from build123d import *

# Parameters (mm, degrees)
SKETCH1_W           = 292.1
SKETCH1_H           = 101.0158
SKETCH1_W_2         = 6.35
SKETCH1_H_2         = 7.62
BOSS_EXTRUDE1_DEPTH = 6
SKETCH2_R           = 11.125
SKETCH2_R_2         = 1.5875
SKETCH2_R_3         = 1.4605
CUT_EXTRUDE1_DEPTH  = 310.132013628
SKETCH3_W           = 7.62
SKETCH3_H           = 6
CUT_EXTRUDE2_DEPTH  = 310.132013628
SKETCH4_W           = 7.62
SKETCH4_H           = 0.35
CUT_EXTRUDE3_DEPTH  = 6
FILLET1_R           = 2.54
SKETCH5_R           = 1.143
CUT_EXTRUDE4_DEPTH  = 310.132013628
SKETCH6_R           = 1.905
SKETCH6_W           = 6.35
SKETCH6_H           = 7.62
CUT_EXTRUDE5_DEPTH  = 310.132013628
SKETCH7_R           = 1.8034
CUT_EXTRUDE6_DEPTH  = 310.132013628
SKETCH8_R           = 1.5875
CUT_EXTRUDE7_DEPTH  = 310.132013628


with BuildPart() as part:
    # Sketch1 → Boss-Extrude1 (new body)
    with BuildSketch(Plane.XY):
        with Locations((146.05, 50.5079)):
            Rectangle(SKETCH1_W, SKETCH1_H)
        with Locations((231.775, 93.7514)):
            Rectangle(SKETCH1_W_2, SKETCH1_H_2, mode=Mode.SUBTRACT)
        with Locations((73.025, 93.7514)):
            Rectangle(SKETCH1_W_2, SKETCH1_H_2, mode=Mode.SUBTRACT)
        with Locations((231.775, 7.2644)):
            Rectangle(SKETCH1_W_2, SKETCH1_H_2, mode=Mode.SUBTRACT)
        with Locations((73.025, 7.2644)):
            Rectangle(SKETCH1_W_2, SKETCH1_H_2, mode=Mode.SUBTRACT)
    extrude(amount=BOSS_EXTRUDE1_DEPTH)

    # Sketch2 → Cut-Extrude1 (cut, through all)
    with BuildSketch(Plane.XY.offset(6)):
        with Locations((271.1, 56.4261)):
            Circle(SKETCH2_R)
        with Locations((255.6, 71.9261)):
            Circle(SKETCH2_R_2)
        with Locations((255.6, 40.9261)):
            Circle(SKETCH2_R_2)
        with Locations((286.6, 40.9261)):
            Circle(SKETCH2_R_2)
        with Locations((286.6, 71.9261)):
            Circle(SKETCH2_R_2)
        with Locations((271.1, 40.9261)):
            Circle(SKETCH2_R_3)
    extrude(amount=-CUT_EXTRUDE1_DEPTH, mode=Mode.SUBTRACT)

    # Sketch3 → Cut-Extrude2 (cut, through all)
    with BuildSketch(Plane.XY.offset(6)):
        with Locations((117.19, 94.5614)):
            Rectangle(SKETCH3_W, SKETCH3_H)
        with Locations((117.19, 6.4544)):
            Rectangle(SKETCH3_W, SKETCH3_H)
        with Locations((28.29, 6.4544)):
            Rectangle(SKETCH3_W, SKETCH3_H)
        with Locations((28.29, 94.5614)):
            Rectangle(SKETCH3_W, SKETCH3_H)
    extrude(amount=-CUT_EXTRUDE2_DEPTH, mode=Mode.SUBTRACT)

    # Sketch4 → Cut-Extrude3 (cut)
    with BuildSketch(Plane.XY.offset(6)):
        with Locations((28.29, 91.3864)):
            Rectangle(SKETCH4_W, SKETCH4_H)
        with Locations((28.29, 9.6294)):
            Rectangle(SKETCH4_W, SKETCH4_H)
        with Locations((117.19, 9.6294)):
            Rectangle(SKETCH4_W, SKETCH4_H)
        with Locations((117.19, 91.3864)):
            Rectangle(SKETCH4_W, SKETCH4_H)
    extrude(amount=-CUT_EXTRUDE3_DEPTH, mode=Mode.SUBTRACT)

    # Fillet1
    fillet1_edges = [part.edges().sort_by_distance(p)[0] for p in [
        (0, 101.0158, 3),
        (292.1, 101.0158, 3),
        (292.1, 0, 3),
        (0, 0, 3),
    ]]
    fillet(fillet1_edges, radius=FILLET1_R)

    # Sketch5 → Cut-Extrude4 (cut, through all)
    with BuildSketch(Plane.XY.offset(6)):
        with Locations((35.306, 39.824852294)):
            Circle(SKETCH5_R)
        with Locations((41.275, 61.190947706)):
            Circle(SKETCH5_R)
    extrude(amount=-CUT_EXTRUDE4_DEPTH, mode=Mode.SUBTRACT)

    # Sketch6 → Cut-Extrude5 (cut, through all)
    with BuildSketch(Plane.XY.offset(6)):
        with Locations((146.4, 96.2533)):
            Circle(SKETCH6_R)
        with Locations((215.9, 96.2533)):
            Circle(SKETCH6_R)
        with Locations((215.9, 4.7625)):
            Circle(SKETCH6_R)
        with Locations((146.4, 4.7625)):
            Circle(SKETCH6_R)
        with Locations((133.7, 93.7514)):
            Rectangle(SKETCH6_W, SKETCH6_H)
        with Locations((133.7, 7.2644)):
            Rectangle(SKETCH6_W, SKETCH6_H)
    extrude(amount=-CUT_EXTRUDE5_DEPTH, mode=Mode.SUBTRACT)

    # Sketch7 → Cut-Extrude6 (cut, through all)
    with BuildSketch(Plane.XY.offset(6)):
        with Locations((16.5679, 94.2114)):
            Circle(SKETCH7_R)
        with Locations((105.4679, 94.2114)):
            Circle(SKETCH7_R)
        with Locations((105.4679, 6.1044)):
            Circle(SKETCH7_R)
        with Locations((16.5679, 6.1044)):
            Circle(SKETCH7_R)
    extrude(amount=-CUT_EXTRUDE6_DEPTH, mode=Mode.SUBTRACT)

    # Sketch8 → Cut-Extrude7 (cut, through all)
    with BuildSketch(Plane.XY.offset(6)):
        with Locations((279.4, 101.0158)):
            Circle(SKETCH8_R)
    extrude(amount=-CUT_EXTRUDE7_DEPTH, mode=Mode.SUBTRACT)


solid = part.part
Geometry check sheet. Reference: the model listing, model coordinates, mm. Coordinates: 2 decimals unless noted, no trailing zeros. Write each loop counter-clockwise with the first axis right and the second up, starting at its lowest first coordinate (ties: lowest second). Pieces come first, ordered by that corner, then holes. Notation, with made-up numbers: (-34.5, 12) -> (17.5, 12) arc R8 ccw to (17.5, 21) -> close; hole circle Ø3 at (21, 33). An arc over 180 degrees is marked (long way). One line per question, with ' | ' between items.
1. Draft check along Y on faces 1 (the flat face through (73, 97.561, 3)), 2 (the flat face through (138, 101.016, 3)), 3 (the flat face through (0, 50, 3)). Enter one of: +Y half, -Y half, draft (parallel to the pull), parting line (faces both ways), or undercut.
Answers:
face 1: undercut | face 2: +Y half | face 3: draft
2. Cross-section at A-A on x = 28. Record the cut outline in (y, z), and give its area (3 significant figures).
Answers:
outline: (0, 0) -> (3.45, 0) -> (3.45, 6) -> (0, 6) -> close; (9.8, 0) -> (91.21, 0) -> (91.21, 6) -> (9.8, 6) -> close; (97.56, 0) -> (101.02, 0) -> (101.02, 6) -> (97.56, 6) -> close | area: 530 mm²
3. Cross-section at B-B on y = 51. Record the cut outline in (x, z), and give its area (3 significant figures).
Answers:
outline: (0, 0) -> (261.39, 0) -> (261.39, 6) -> (0, 6) -> close; (280.81, 0) -> (292.1, 0) -> (292.1, 6) -> (280.81, 6) -> close | area: 1,640 mm²
4. Thickness scan on probe 1 along Y at (x, z) = (72, 4.1); probe 2 along X at (y, z) = (9, 0.7) (3 decimals); probe 3 along X at (y, z) = (60.5, 0.95). Record the ranges inside material, lowest first. Write a range as from..to.
Answers:
probe 1: y = 0..3.45, 11.07..89.94, 97.56..101.02 | probe 2: x = 0..24.48, 32.1..69.85, 76.2..113.38, 121..130.525, 136.875..228.6, 234.95..292.1 | probe 3: x = 0..40.36, 42.19..260.75, 281.45..292.1
5. Cross-section at C-C on z = 2.8. State how many separate pieces and enclosed holes the cut face has, and give its area (3 significant figures).
Answers:
separate pieces: 1 | enclosed holes: 26 | area: 28,500 mm²
